Autodesk Inventor part; units mm, degrees
ref_plane "YZ Plane" through (0, 0, 0) normal (1, 0, 0) x (0, 1, 0)
ref_plane "XZ Plane" through (0, 0, 0) normal (0, 1, 0) x (-1, 0, 0)
ref_plane "XY Plane" through (0, 0, 0) normal (0, 0, 1) x (1, 0, 0)
sketch "Sketch1" plane through (0, 0, 0) normal (0, 0, 1) x (1, 0, 0)
  circle A0 centre (0, 0) radius 9.525
  dimension "d0" = 19.05
extrude "Extrusion1" add sketch "Sketch1" along normal blind 148.0058
sketch "Sketch2" plane through (0, 0, 148.0058) normal (0, 0, 1) x (1, 0, 0)
  point P0 (0, 0)
  point P1 (0, 0)
sketch "Sketch3" plane through (0, 0, 0) normal (0, 0, -1) x (-1, 0, 0)
  point P0 (0, 0)
  point P1 (0, 0)
hole "Hole1" at (0, 0, 0) direction (0, 0, 1) diameter 4.9784 depth 19.05 tip angle 118
hole "Hole2" at (0, 0, 148.0058) direction (0, 0, -1) diameter 4.9784 depth 19.05 tip angle 118
properties part number "Plate Spacer" material "Aluminum 6061"
Work out the finished part from the listing and answer in its coordinate system (mm). A direction names the side the tool comes from. Give positions to 0.01 mm unless a question says otherwise; leave off trailing zeros. Write each loop counter-clockwise with the first axis right and the second up, starting at its lowest first coordinate (ties: lowest second). Pieces come first, ordered by that corner, then holes.
Q1. The part is cut by section C-C on x = 7.5. Give the vertices of the cut face in (y, z), and give its area (3 significant figures).
Answer:
outline: (-5.87, 0) - (5.87, 0) - (5.87, 148.01) - (-5.87, 148.01) - close
area: 1,740 mm2
Q2. For a pull along Y with two mould halves and no side action, classify faces 1 (the face through (2, -2, 0)), 2 (the face through (-7.559, 5.796, 72.967)), 3 (the face through (-0.748, 2.374, 9.658)) as released by +Y, released by -Y, zero draft, split by the parting line, or undercut.
Answer:
face 1: zero draft
face 2: split by the parting line
face 3: undercut
Q3. The part is cut by section B-B on y = 4.5. Give the vertices of the cut face in (x, z), and give its area (3 significant figures).
Answer:
outline: (-8.39, 0) - (8.39, 0) - (8.39, 148.01) - (-8.39, 148.01) - close
area: 2,490 mm2
Q4. Straight lines are drawn through the part: L1, parallel to Y at x = 0, z = 13 (3 decimals); L2, parallel to Y at x = -1.25, z = 136; L3, parallel to X at y = -2.25, z = 130.5. For each, find the intervals that lie inside material, in ascending order.
Answer:
L1: y = -9.525 to -2.489, 2.489 to 9.525
L2: y = -9.44 to -2.15, 2.15 to 9.44
L3: x = -9.26 to -1.06, 1.06 to 9.26
Q5. Given pin 1 (4 mm diameter, centred on y = -5, z = 26, fed in from -X); pin 2 (5 mm diameter, centred on x = -7, z = 60.5, fed in from -Y) (3 decimals), each flat-ended and moving along its own axis, determine where each tip first touches the part or whether it passes through.
Answer:
pin 1: stops at x = -9.04
pin 2: stops at y = -8.395
Q6. The part is cut by section A-A on z = 108. Give the vertices of the cut face in (x, y) (3 decimals).
Answer:
outline: circle Ø19.05 at (0, 0)
Q7. A tool of negligible diameter and unlimited length cuts with its end or side. For faces 4 (the face through (-0.4, -0.1, 20.3)), 5 (the face through (-0.748, -2.374, 138.347)), from which of +Z, -Z, +X, -X, +Y, -Y can it reach the whole face along a straight path? Write none if from no direction.
Answer:
face 4: -Z
face 5: +Z
